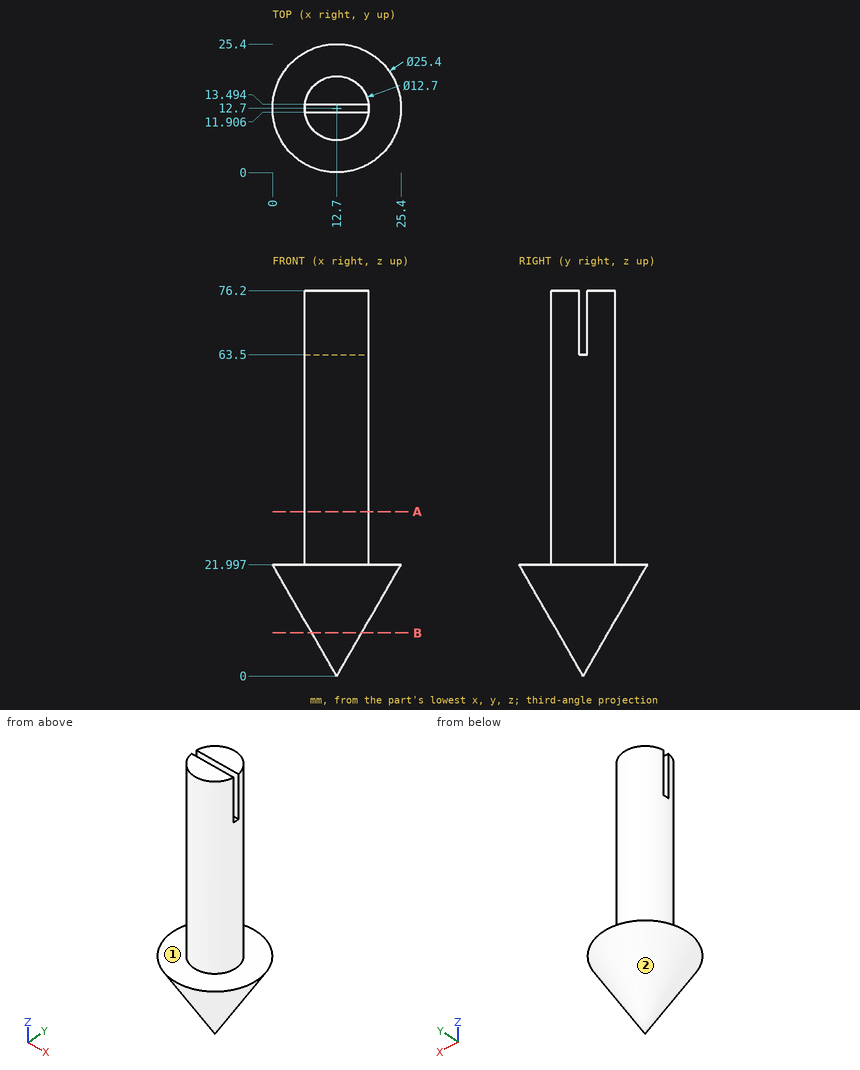
Study the drawing (mm; zero at the part's minimum x, y, z) and answer. A direction names the side the tool comes from. Coordinates: 2 decimals unless noted, no trailing zeros. Write each loop counter-clockwise with the first axis right and the second up, starting at its lowest first coordinate (ties: lowest second). Pieces come first, ordered by that corner, then holes. Notation, with made-up numbers: (19, 32) - (53, 32) arc R16 cw to (53, 52) - close; hole circle Ø8 at (2, 5.25). An arc over 180 degrees is marked (long way). Return JSON: item names as keys, results as strings. Group by question number.
1. Given pin 1 (6 mm diameter, centred on y = 13.5, z = 16, fed in from -X); pin 2 (6.5 mm diameter, centred on x = 15, z = 72, fed in from +Y); pin 3 (4 mm diameter, centred on x = 13.5, z = 39.5, fed in from -Y); pin 4 (6 mm diameter, centred on y = 22.5, z = 34, fed in from -X), each flat-ended and moving along its own axis, determine where each tip first touches the part or whether it passes through.
2. A cutting plane is placed at A-A, the plane z = 32.5. Determine the outline of the cut face in (x, y), plus the area to 3 significant figures.
3. A cutting plane is placed at B-B, the plane z = 8.5. Determine the outline of the cut face in (x, y) (1 decimal).
4. Which of the six approach directions +Z, -Z, +X, -X, +Y, -Y give full straight-line access (tool end or side, diameter ignored) to the marked faces 1 and 2?
5. Straight lines are drawn through the part: L1, parallel to Y at x = 12.75, z = 68; L2, parallel to Z at x = 16.75, y = 17.25; L3, parallel to Z at x = 1.75, y = 8.75 (1 decimal). For each, find the intervals that lie inside material, in ascending order.
Ans:
{
 "1": {"pin 1": "x = 1.75", "pin 2": "y = 19.05", "pin 3": "y = 6.35", "pin 4": "through"},
 "2": {"outline": "circle Ø12.7 at (12.7, 12.7)", "area": "127 mm²"},
 "3": {"outline": "circle Ø9.8 at (12.7, 12.7)"},
 "4": {"face 1": "+Z", "face 2": "-Z"},
 "5": {"L1": "6.35 to 11.91, 13.49 to 19.05", "L2": "10.55 to 76.2", "L3": "20.2 to 22"}
}
